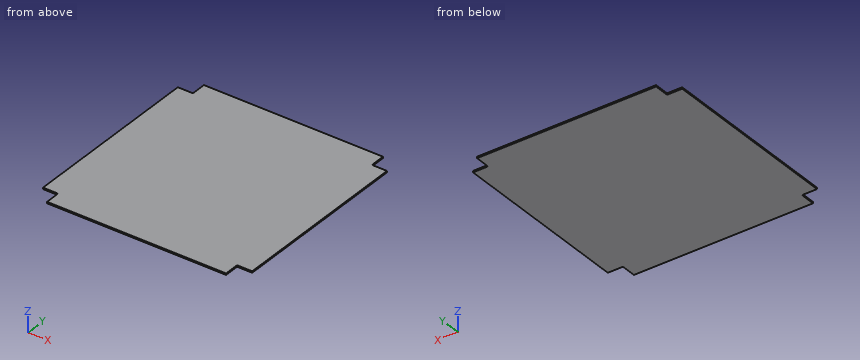
from build123d import *

# Parameters (mm, degrees)
BOSS_EXTRUDE1_DEPTH = 3


with BuildPart() as part:
    # Sketch1 → Boss-Extrude1 (new body)
    with BuildSketch(Plane.XY):
        with BuildLine():
            Line((215, -189), (215, 189))
            Line((215, 189), (186, 189))
            ThreePointArc((186, 189), (184.585786438, 189.585786438), (184, 191))
            Line((184, 191), (184, 220))
            Line((184, 220), (-184, 220))
            Line((-184, 220), (-184, 191))
            ThreePointArc((-184, 191), (-184.585786438, 189.585786438), (-186, 189))
            Line((-186, 189), (-215, 189))
            Line((-215, 189), (-215, -189))
            Line((-215, -189), (-186, -189))
            ThreePointArc((-186, -189), (-184.585786438, -189.585786438), (-184, -191))
            Line((-184, -191), (-184, -220))
            Line((-184, -220), (184, -220))
            Line((184, -220), (184, -191))
            ThreePointArc((184, -191), (184.585786438, -189.585786438), (186, -189))
            Line((186, -189), (215, -189))
        make_face()
    extrude(amount=BOSS_EXTRUDE1_DEPTH)


solid = part.part
Work out the finished part from the listing and answer in its coordinate system (mm). Give positions to 0.01 mm unless a question says otherwise; leave off trailing zeros. Loops run counter-clockwise (first coordinate to the right, second up) from the corner with the lowest first, then second, coordinate; pieces in that order, holes last. Notation, with made-up numbers: (20.25, 15.25) - (54.25, 15.25) arc R16 ccw to (54.25, 42.25) - close; hole circle Ø11 at (9, 25.5). An arc over 180 degrees is marked (long way). Answer in a Markdown table with one row per item.
(1) Consider L1, parallel to Y at x = -195, z = 1.4. Determine where the line is inside the solid, lowest interval first. Write a range as [from, to].
Results list:
| item | result |
|---|---|
| L1 | y = [-189, 189] |
(2) Section A-A (z = 1.3) is taken. Give the vertices of the cut face in (x, y), and give its area (3 significant figures).
Results list:
| item | result |
|---|---|
| outline | (-215, -189) - (-186, -189) arc R2 cw to (-184, -191) - (-184, -220) - (184, -220) - (184, -191) arc R2 cw to (186, -189) - (215, -189) - (215, 189) - (186, 189) arc R2 cw to (184, 191) - (184, 220) - (-184, 220) - (-184, 191) arc R2 cw to (-186, 189) - (-215, 189) - close |
| area | 185,000 mm² |
(3) Flat-ended cylindrical pins translate along their axes: pin 1 Ø0.9 at (y, z) = (201, 1) entering from +X; pin 2 Ø0.9 at (y, z) = (-206.5, 2) entering from -X; pin 3 Ø1.5 at (x, z) = (-198.5, 1) entering from +Y. Find the tip coordinate at first contact, or state that the pin passes through.
Results list:
| item | result |
|---|---|
| pin 1 | stops at x = 184 |
| pin 2 | stops at x = -184 |
| pin 3 | stops at y = 189 |
